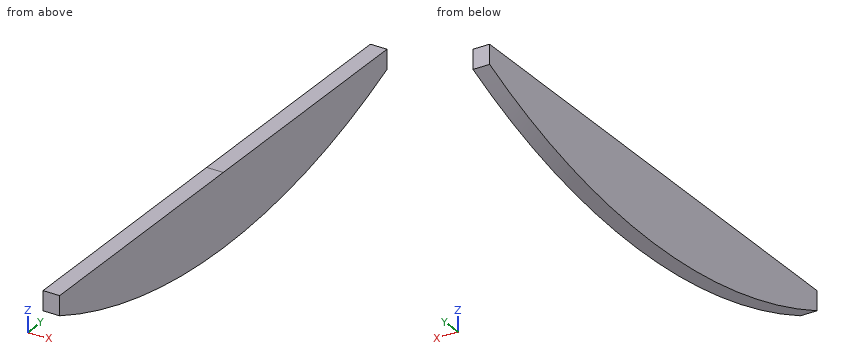
```python
from build123d import *

# Parameters (mm, degrees)
F0_DEPTH = 38.1


with BuildPart() as f0:
    # F2 (on Right) → F0 (new body)
    with BuildSketch(Plane.YZ):
        with BuildLine():
            Line((0, 0), (-590.55, 0))
            Line((-590.55, 0), (-590.55, -44.45))
            ThreePointArc((-590.55, -44.45), (0, -166.226991), (590.55, -44.45))
            Line((590.55, -44.45), (590.55, 0))
            Line((590.55, 0), (0.01061, 0))
            Line((0.01061, 0), (0.01061, -0.003131))
            Line((0.01061, -0.003131), (0, 0))
        make_face()
    extrude(amount=F0_DEPTH)


solid = f0.part
```
Input: part model. Units: mm. Frame: model coordinates. Give positions to 0.01 mm unless a question says otherwise; leave off trailing zeros. Loops run counter-clockwise (first coordinate to the right, second up) from the corner with the lowest first, then second, coordinate; pieces in that order, holes last.
1) Section query C-C on y = 289. Return the cut outline in (x, z), and give its area (3 significant figures).
A:
outline: (0, -137.99) - (38.1, -137.99) - (38.1, 0) - (0, 0) - close
area: 5,260 mm2
2) Section query B-B on z = -145. Return the cut outline in (x, y).
A:
outline: (0, -250.85) - (38.1, -250.85) - (38.1, 250.85) - (0, 250.85) - close
3) Line query: L1, parallel to Z at x = 30, y = -10; L2, parallel to Z at x = 11, y = 504; L3, parallel to Y at x = 5.5, z = -50.5. Output: solid intervals per line, ascending.
A:
L1: z = -166.19 to 0
L2: z = -78.57 to 0
L3: y = -576.3 to 576.3
